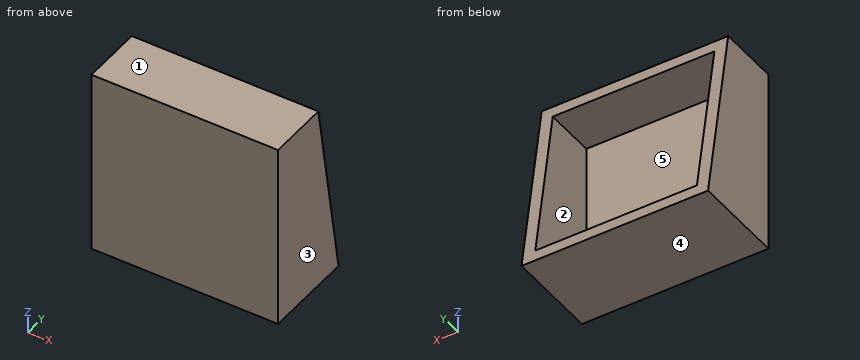
```python
from build123d import *

# Parameters (mm, degrees)
ESQUISSE1_W             = 300
ESQUISSE1_H             = 150
BOSS_EXTRU_1_DEPTH      = 300
ENL_V_MAT_EXTRU_5_DEPTH = 300
COQUE2_T                = -20


with BuildPart() as part:
    # Esquisse1 → Boss.-Extru.1 (new body)
    with BuildSketch(Plane.XY):
        with Locations((150, 75)):
            Rectangle(ESQUISSE1_W, ESQUISSE1_H)
    extrude(amount=BOSS_EXTRU_1_DEPTH)

    # Esquisse5 → Enlèv. mat.-Extru.5 (cut)
    with BuildSketch(Plane(origin=(300, 0, 0), x_dir=(0, 0, -1), z_dir=(1, 0, 0))):
        Polygon((0, 150), (-300, 100), (-300, 150), align=None)
    extrude(amount=-ENL_V_MAT_EXTRU_5_DEPTH, mode=Mode.SUBTRACT)

    # Coque2
    coque2_openings = [part.faces().sort_by_distance(p)[0] for p in [
        (150, 125, 150),
    ]]
    offset(amount=COQUE2_T, openings=coque2_openings, kind=Kind.INTERSECTION)


solid = part.part
```
Model file for the job. Use its own axes, mm. Face numbers are marked on the shaded views. A direction names the side the tool comes from. Coordinates: 2 decimals unless noted, no trailing zeros. Loops run counter-clockwise (first coordinate to the right, second up) from the corner with the lowest first, then second, coordinate; pieces in that order, holes last. Notation, with made-up numbers: (9, -15.75) -> (44, -15.75) arc R30 ccw to (44, 20.25) -> close; hole circle Ø2 at (-6.75, -28). An arc over 180 degrees is marked (long way). Answer as a JSON object with one key per item and string values.
Q1. 3-axis set-ups, long thin cutter, end or side, ignore diameter. For the marked faces 4 and 5: which of +Z, -Z, +X, -X, +Y, -Y reach the whole face in a straight line?
Report:
{"face 4": "-Z, +X, -X, +Y, -Y", "face 5": "+Y"}
Q2. Probe probe 1 along Z at (x, y) = (44, 24.5); probe 2 along Z at (x, y) = (122, 131.5). List the from-to ranges inside material, lowest first.
Report:
{"probe 1": "z = 0 to 20, 280 to 300", "probe 2": "z = 0 to 20"}
Q3. Flat gauge pin, fed straight in: P1, Ø1.5, axis at x = 104, z = 229, coming from the +Y side. Where does the tip first touch, or does it go through?
Report:
{"P1": "stops at y = 20"}
Q4. Pull direction X, two halves, no side cores. Call the marked faces 1, 2 and 3: released by +X, released by -X, zero draft, split by the parting line, or undercut.
Report:
{"face 1": "zero draft", "face 2": "undercut", "face 3": "released by +X"}
Q5. Cut at B-B (z = 112.5). List the corners of the cut face in (x, y).
Report:
{"outline": "(0, 0) -> (300, 0) -> (300, 131.25) -> (280, 131.25) -> (280, 20) -> (20, 20) -> (20, 131.25) -> (0, 131.25) -> close"}
Q6. Cut at C-C (y = 118.5). List the corners of the cut face in (x, z).
Report:
{"outline": "(0, 0) -> (300, 0) -> (300, 189) -> (280, 189) -> (280, 20) -> (20, 20) -> (20, 189) -> (0, 189) -> close"}
Q7. Cut at A-A (y = 43). List the corners of the cut face in (x, z).
Report:
{"outline": "(0, 0) -> (300, 0) -> (300, 300) -> (0, 300) -> close; hole (20, 20) -> (280, 20) -> (280, 280) -> (20, 280) -> close"}
